```python
from build123d import *

# Parameters (mm, degrees)
IZIM1_W                     = 10
IZIM1_H                     = 10
Y_KSEKLIK_EKSTR_ZYON1_DEPTH = 10
KES_EKSTR_ZYON1_DEPTH       = 10
IZIM3_W                     = 9.22702718
IZIM3_H                     = 8.892036637
KES_EKSTR_ZYON2_DEPTH       = 10
KES_EKSTR_ZYON3_DEPTH       = 10
IZIM6_R                     = 1.5
KES_EKSTR_ZYON4_DEPTH       = 10


with BuildPart() as part:
    # Çizim1 → Yükseklik-Ekstrüzyon1 (new body)
    with BuildSketch(Plane(origin=(0, 0, 0), x_dir=(1, 0, 0), z_dir=(0, 1, 0))):
        with Locations((-23.640485452, -27.285638146)):
            Rectangle(IZIM1_W, IZIM1_H)
    extrude(amount=Y_KSEKLIK_EKSTR_ZYON1_DEPTH)

    # Çizim2 → Kes-Ekstrüzyon1 (cut)
    with BuildSketch(Plane(origin=(0, 10, 0), x_dir=(1, 0, 0), z_dir=(0, 1, 0))):
        Polygon((-28.640485452, -22.285638146), (-18.640485452, -22.285638146), (-28.640485452, -32.285638146), align=None)
    extrude(amount=-KES_EKSTR_ZYON1_DEPTH, mode=Mode.SUBTRACT)

    # Çizim3 → Kes-Ekstrüzyon2 (cut)
    with BuildSketch(Plane(origin=(0, 10, 0), x_dir=(1, 0, 0), z_dir=(0, 1, 0))):
        with Locations((-24.668212605, -26.425406266)):
            Rectangle(IZIM3_W, IZIM3_H)
    extrude(amount=-KES_EKSTR_ZYON2_DEPTH, mode=Mode.SUBTRACT)

    # Çizim5 → Kes-Ekstrüzyon3 (cut)
    with BuildSketch(Plane.ZY.offset(20.054699015)):
        with BuildLine():
            ThreePointArc((28.785638146, 5), (27.970743901, 6.334402527), (26.411464673, 6.218942467))
            Line((26.411464673, 6.218942467), (28.15981162, 3.781057533))
            ThreePointArc((28.15981162, 3.781057533), (28.620040674, 4.314894245), (28.785638146, 5))
        make_face()
        with BuildLine():
            Line((28.15981162, 3.781057533), (26.411464673, 6.218942467))
            ThreePointArc((26.411464673, 6.218942467), (26.066695679, 4.125826527), (28.15981162, 3.781057533))
        make_face()
    extrude(amount=-KES_EKSTR_ZYON3_DEPTH, mode=Mode.SUBTRACT)

    # Çizim6 → Kes-Ekstrüzyon4 (cut)
    with BuildSketch(Plane(origin=(0, 0, 30.871424584), x_dir=(-1, 0, 0), z_dir=(0, 0, -1))):
        with Locations((23.640485452, 5)):
            Circle(IZIM6_R)
    extrude(amount=-KES_EKSTR_ZYON4_DEPTH, mode=Mode.SUBTRACT)


solid = part.part
```
Build history of the part. All positions in model axes, mm. A direction names the side the tool comes from. Give positions to 0.01 mm unless a question says otherwise; leave off trailing zeros. Loops run counter-clockwise (first coordinate to the right, second up) from the corner with the lowest first, then second, coordinate; pieces in that order, holes last. Notation, with made-up numbers: (28, 30) -> (36, 30) arc R29 cw to (36, 69) -> close; hole circle Ø9 at (9, 66). An arc over 180 degrees is marked (long way). One line per question, with ' | ' between items. Start each with the question number.
1) 3-axis set-ups, long thin cutter, end or side, ignore diameter. For faces 4 (the flat face through (-21.4, 10, 31.3)), 5 (the flat face through (-25.3, 5.1, 30.871)): which of +Z, -Z, +X, -X, +Y, -Y reach the whole face in a straight line?
2) Cut at A-A (x = -23.75). Give the cut face in (y, z), plus the area to 3 significant figures.
3) Two-plate mould, pull along Y, no slides. Class faces 1 (the flat face through (-20.055, 5, 29)), 2 (the flat face through (-21.4, 0, 31.3)), 3 (the cylindrical face through (-25.07, 5.45, 31.57)): released by +Y, released by -Y, zero draft, split by the parting line, or undercut.
4) Cut at B-B (y = 5.25). Give the cut face in (x, z).
5) Pin check, flat tips, straight feed: pin 1 (3.5 mm diameter, centred on y = 7, z = 28, fed in from -X); pin 2 (3 mm diameter, centred on x = -22, z = 28.5, fed in from -Y); pin 3 (3.5 mm diameter, centred on x = -23.64, y = 5, fed in from -Z). Stop position of each tip, or through.
6) Cut at C-C (z = 26.25). Give the cut face in (x, y).
7) Cut at D-D (z = 24.25). Give the cut face in (x, y).
8) Probe L1, parallel to Z at x = -20.5, y = 1; L2, parallel to X at y = 6.5, z = 27.75; L3, parallel to Y at x = -19.5, z = 27. List the from-to ranges inside material, lowest first.
Return value:
1) face 4: +Z, -Z, +X, -X, +Y | face 5: -Z, -X, +Y, -Y
2) outline: (0, 30.87) -> (3.5, 30.87) -> (3.5, 32.29) -> (0, 32.29) -> close; (6.5, 30.87) -> (10, 30.87) -> (10, 32.29) -> (6.5, 32.29) -> close | area: 9.91 mm^2
3) face 1: zero draft | face 2: released by -Y | face 3: undercut
4) outline: (-28.64, 32.29) -> (-27.23, 30.87) -> (-25.12, 30.87) -> (-25.12, 32.29) -> close; (-22.16, 30.87) -> (-20.05, 30.87) -> (-20.05, 28.76) -> (-18.64, 28.76) -> (-18.64, 32.29) -> (-22.16, 32.29) -> close; (-20.05, 23.7) -> (-18.64, 22.29) -> (-18.64, 25.81) -> (-20.05, 25.81) -> close
5) pin 1: x = -20.05 | pin 2: through | pin 3: z = 30.87
6) outline: (-20.05, 0) -> (-18.64, 0) -> (-18.64, 3.91) -> (-20.05, 3.91) -> close; (-20.05, 6.09) -> (-18.64, 6.09) -> (-18.64, 10) -> (-20.05, 10) -> close
7) outline: (-20.05, 0) -> (-18.64, 0) -> (-18.64, 10) -> (-20.05, 10) -> close
8) L1: 30.87 to 32.29 | L2: -20.05 to -18.64 | L3: 0 to 3.53, 6.47 to 10
